from build123d import *

# Parameters (mm, degrees)
SKETCH1_W           = 194
SKETCH1_H           = 40
BOSS_EXTRUDE1_DEPTH = 10
SKETCH3_W           = 6
SKETCH3_H           = 6
SKETCH3_W_2         = 26
SKETCH3_H_2         = 8
CUT_EXTRUDE1_DEPTH  = 11
CHAMFER1_SIZE       = 1
CHAMFER2_SIZE       = 1
SKETCH4_W           = 5
SKETCH4_H           = 5
CUT_EXTRUDE2_DEPTH  = 7
CHAMFER3_SIZE       = 1
CUT_EXTRUDE4_DEPTH  = 195
CUT_EXTRUDE5_DEPTH  = 41


with BuildPart() as part:
    # Sketch1 → Boss-Extrude1 (new body)
    with BuildSketch(Plane(origin=(0, 0, 0), x_dir=(1, 0, 0), z_dir=(0, 1, 0))):
        Rectangle(SKETCH1_W, SKETCH1_H)
    extrude(amount=BOSS_EXTRUDE1_DEPTH)

    # Sketch3 → Cut-Extrude1 (cut, through all)
    with BuildSketch(Plane(origin=(0, 10, 0), x_dir=(1, 0, 0), z_dir=(0, 1, 0))):
        with Locations((-88, 2)):
            Rectangle(SKETCH3_W, SKETCH3_H)
        with Locations((-75.7, 2)):
            Rectangle(SKETCH3_W, SKETCH3_H)
        with Locations((-63.4, 2)):
            Rectangle(SKETCH3_W, SKETCH3_H)
        with Locations((-51.1, 2)):
            Rectangle(SKETCH3_W, SKETCH3_H)
        with Locations((-38.8, 2)):
            Rectangle(SKETCH3_W, SKETCH3_H)
        with Locations((-26.5, 2)):
            Rectangle(SKETCH3_W, SKETCH3_H)
        with Locations((-14.2, 2)):
            Rectangle(SKETCH3_W, SKETCH3_H)
        with Locations((-1.9, 2)):
            Rectangle(SKETCH3_W, SKETCH3_H)
        with Locations((10.4, 2)):
            Rectangle(SKETCH3_W, SKETCH3_H)
        with Locations((22.7, 2)):
            Rectangle(SKETCH3_W, SKETCH3_H)
        with Locations((35, 2)):
            Rectangle(SKETCH3_W, SKETCH3_H)
        with Locations((47.3, 2)):
            Rectangle(SKETCH3_W, SKETCH3_H)
        with Locations((-88, 12)):
            Rectangle(SKETCH3_W, SKETCH3_H)
        with Locations((-88, -8)):
            Rectangle(SKETCH3_W, SKETCH3_H)
        with Locations((-12, -12.5)):
            Rectangle(SKETCH3_W_2, SKETCH3_H_2)
    extrude(amount=-CUT_EXTRUDE1_DEPTH, mode=Mode.SUBTRACT)

    # Chamfer1
    chamfer1_edges = [part.edges().sort_by_distance(p)[0] for p in [
        (-26.5, 10, -5),
        (-29.5, 10, -2),
        (-14.2, 10, 1),
        (-11.2, 10, -2),
        (-14.2, 10, -5),
        (-17.2, 10, -2),
        (-1.9, 10, 1),
        (1.1, 10, -2),
        (-1.9, 10, -5),
        (-4.9, 10, -2),
        (10.4, 10, 1),
        (13.4, 10, -2),
        (10.4, 10, -5),
        (7.4, 10, -2),
        (1, 10, 12.5),
        (-12, 10, 8.5),
        (-25, 10, 12.5),
        (-12, 10, 16.5),
        (-88, 10, -9),
        (-85, 10, -12),
        (-88, 10, -15),
        (-91, 10, -12),
        (22.7, 10, 1),
        (25.7, 10, -2),
        (22.7, 10, -5),
        (19.7, 10, -2),
        (35, 10, 1),
        (38, 10, -2),
        (35, 10, -5),
        (32, 10, -2),
        (47.3, 10, 1),
        (47.3, 10, -5),
        (44.3, 10, -2),
        (-88, 10, 11),
        (-85, 10, 8),
        (-88, 10, 5),
        (-91, 10, 8),
        (-85, 10, -2),
        (-88, 10, -5),
        (-91, 10, -2),
        (-88, 10, 1),
        (-75.7, 10, 1),
        (-72.7, 10, -2),
        (-75.7, 10, -5),
        (-78.7, 10, -2),
        (-63.4, 10, 1),
        (-60.4, 10, -2),
        (-63.4, 10, -5),
        (-66.4, 10, -2),
        (-51.1, 10, 1),
        (-48.1, 10, -2),
        (-51.1, 10, -5),
        (-54.1, 10, -2),
        (-38.8, 10, 1),
        (-35.8, 10, -2),
        (-38.8, 10, -5),
        (-41.8, 10, -2),
        (-26.5, 10, 1),
        (-23.5, 10, -2),
    ]]
    chamfer(chamfer1_edges, length=CHAMFER1_SIZE)

    # Chamfer2
    chamfer2_edges = [part.edges().sort_by_distance(p)[0] for p in [
        (-14.2, 0, 1),
        (-17.2, 0, -2),
        (-14.2, 0, -5),
        (-11.2, 0, -2),
        (-1.9, 0, 1),
        (-4.9, 0, -2),
        (-1.9, 0, -5),
        (1.1, 0, -2),
        (10.4, 0, 1),
        (7.4, 0, -2),
        (10.4, 0, -5),
        (13.4, 0, -2),
        (1, 0, 12.5),
        (-12, 0, 16.5),
        (-25, 0, 12.5),
        (-12, 0, 8.5),
        (-88, 0, -9),
        (-91, 0, -12),
        (-88, 0, -15),
        (-85, 0, -12),
        (22.7, 0, 1),
        (19.7, 0, -2),
        (22.7, 0, -5),
        (25.7, 0, -2),
        (35, 0, 1),
        (32, 0, -2),
        (35, 0, -5),
        (38, 0, -2),
        (47.3, 0, 1),
        (44.3, 0, -2),
        (47.3, 0, -5),
        (50.3, 0, -2),
        (-88, 0, 11),
        (-91, 0, 8),
        (-88, 0, 5),
        (-85, 0, 8),
        (-85, 0, -2),
        (-88, 0, 1),
        (-91, 0, -2),
        (-88, 0, -5),
        (0, 0, 20),
        (-97, 0, 0),
        (0, 0, -20),
        (97, 0, 0),
        (-75.7, 0, 1),
        (-78.7, 0, -2),
        (-75.7, 0, -5),
        (-72.7, 0, -2),
        (-63.4, 0, 1),
        (-66.4, 0, -2),
        (-63.4, 0, -5),
        (-60.4, 0, -2),
        (-51.1, 0, 1),
        (-54.1, 0, -2),
        (-51.1, 0, -5),
        (-48.1, 0, -2),
        (-38.8, 0, 1),
        (-41.8, 0, -2),
        (-38.8, 0, -5),
        (-35.8, 0, -2),
        (-26.5, 0, 1),
        (-29.5, 0, -2),
        (-26.5, 0, -5),
        (-23.5, 0, -2),
    ]]
    chamfer(chamfer2_edges, length=CHAMFER2_SIZE)

    # Sketch4 → Cut-Extrude2 (cut)
    with BuildSketch(Plane(origin=(0, 10, 0), x_dir=(1, 0, 0), z_dir=(0, 1, 0))):
        with Locations((53.8, 2)):
            Rectangle(SKETCH4_W, SKETCH4_H)
        Polygon((56.3, 12.5), (56.3, 4.5), (56.3, -0.5), (56.3, -7.5), (86.3, -7.5), (86.3, 12.5), align=None)
    extrude(amount=-CUT_EXTRUDE2_DEPTH, mode=Mode.SUBTRACT)

    # Chamfer3
    chamfer3_edges = [part.edges().sort_by_distance(p)[0] for p in [
        (53.8, 10, -4.5),
        (71.3, 10, -12.5),
        (86.3, 10, -2.5),
        (53.8, 10, 0.5),
        (56.3, 10, 4),
        (71.3, 10, 7.5),
        (56.3, 10, -8.5),
    ]]
    chamfer(chamfer3_edges, length=CHAMFER3_SIZE)

    # Sketch6 → Cut-Extrude4 (cut, through all)
    with BuildSketch(Plane.ZY.offset(97)):
        Polygon((-20, 5), (-20, 3), (-19, 4), align=None)
        Polygon((19, 4), (20, 5), (20, 3), align=None)
    extrude(amount=-CUT_EXTRUDE4_DEPTH, mode=Mode.SUBTRACT)

    # Sketch7 → Cut-Extrude5 (cut, through all)
    with BuildSketch(Plane.XY.offset(20)):
        Polygon((-97, 5), (-96, 4), (-97, 3), align=None)
        Polygon((96, 4), (97, 3), (97, 5), align=None)
    extrude(amount=-CUT_EXTRUDE5_DEPTH, mode=Mode.SUBTRACT)


solid = part.part
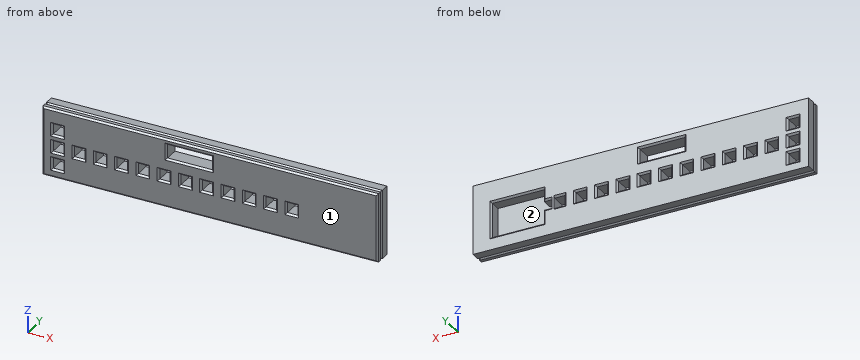
Geometry check sheet. Reference: the model listing, model coordinates, mm. Face numbers are marked on the shaded views. Coordinates: 2 decimals unless noted, no trailing zeros. Order: outer loops, then holes, each group sorted by start corner. A loop starts at its lowest first (then second) coordinate and runs counter-clockwise, first axis right, second up. Notation, with made-up numbers: (-20, -38) -> (27, -38) arc R23 ccw to (27, -29) -> close; hole circle Ø10 at (78, -21). An arc over 180 degrees is marked (long way). Use a Markdown table: item, result. Add a question column.
1. Mould release check, pull along Z, two halves, no side actions. Record for the marked faces 1 and 2: pulls with the +Z half, pulls with the -Z half, needs draft (parallel to the pull), parting line crosses it, or undercut.
2. Material ranges on L1, parallel to Z at x = 0, y = 6.25; L2, parallel to X at y = 9, z = 13; L3, parallel to X at y = 2.75, z = -10.5, recorded low to high.
3. Go/stop test with flat-tipped pins: pin 1 Ø1 at (x, y) = (-9, 4) entering from -Z; pin 2 Ø1.8 at (y, z) = (4, -2) entering from -X; pin 3 Ø1.8 at (x, y) = (-62, 4) entering from -Z. Record where each tip stops, or that it passes through.
4. Cross-section at A-A (x = 35). Enter the section's corners in (y, z), and give its area (3 significant figures).
Filled sheet:
| question | item | result |
|---|---|---|
| 1 | face 1 | needs draft |
| 1 | face 2 | undercut |
| 2 | L1 | -20 to -5, 1 to 8.5, 16.5 to 20 |
| 2 | L2 | -97 to -25, 1 to 97 |
| 2 | L3 | -97 to -91, -85 to 97 |
| 3 | pin 1 | z = -19.5 |
| 3 | pin 2 | x = -96.9 |
| 3 | pin 3 | z = -19.9 |
| 4 | outline | (0, -19) -> (1, -20) -> (3, -20) -> (4, -19) -> (5, -20) -> (10, -20) -> (10, -6) -> (9, -5) -> (1, -5) -> (0, -6) -> close; (0, 2) -> (1, 1) -> (9, 1) -> (10, 2) -> (10, 20) -> (5, 20) -> (4, 19) -> (3, 20) -> (1, 20) -> (0, 19) -> close |
| 4 | area | 335 mm2 |
